Work out the finished part from the listing and answer in its coordinate system (mm). A direction names the side the tool comes from. Coordinates: 2 decimals unless noted, no trailing zeros. Order: outer loops, then holes, each group sorted by start corner. A loop starts at its lowest first (then second) coordinate and runs counter-clockwise, first axis right, second up. Notation, with made-up numbers: (76.25, 24.25) - (108.25, 24.25) arc R12 cw to (108.25, 40.25) - close; hole circle Ø4 at (54.5, 45). An arc over 180 degrees is marked (long way). Answer as a JSON object with one key per item and string values. Group by question number.
1) Find the intervals of material crossed by line 1 along X through (y, z) = (1.5, 14.75); line 2 along X through (y, z) = (7.25, 14.25); line 3 along Y through (x, z) = (15.5, 3), in increasing order.
2) Section B-B (x = 12.5) is taken. Give the vertices of the cut face in (y, z).
3) A tool of negligible diameter and unlimited length cuts with its end or side. For faces 5 (the face through (4.5, 2.2, 19.5)), 6 (the face through (21.6, 14.3, 0.7)), 7 (the face through (14, 13, 14)), from which of +Z, -Z, +X, -X, +Y, -Y can it reach the whole face along a straight path? Write none if from no direction.
4) The mould has two halves that part along Z. Classify faces 1 (the face through (18.7, 7.7, 0.5)), 2 (the face through (2.5, 0.5, 19.5)), 3 (the face through (19.2, 7, 10)), 4 (the face through (7.9, 14.2, 9.9)): released by +Z, released by -Z, zero draft, split by the parting line, or undercut.
5) Each of these flat-tipped pins is pushed along its axis until it touches: P1, Ø2.5, axis at y = 8, z = 6.5, coming from the +X side; P2, Ø4, axis at x = 14, z = 8.5, coming from the +Y side; P3, Ø4, axis at y = 11, z = 18, coming from the -X side; P4, Ø9, axis at x = 11.5, z = 9, coming from the -Y side. Where does it stop, or does it pass through?
Autodesk Inventor part; units mm, degrees
ref_plane "YZ Plane" through (0, 0, 0) normal (1, 0, 0) x (0, 1, 0)
ref_plane "XZ Plane" through (0, 0, 0) normal (0, 1, 0) x (-1, 0, 0)
ref_plane "XY Plane" through (0, 0, 0) normal (0, 0, 1) x (1, 0, 0)
sketch "Base Sketch" plane through (0, 0, 0) normal (0, 0, 1) x (1, 0, 0)
  line L0 (0, 0) -> (5, 0)
  line L1 (5, 0) -> (5, 3)
  line L2 (5, 3) -> (8, 6)
  line L3 (8, 6) -> (19.2, 6)
  line L4 (22.2, 15) -> (0, 15)
  line L5 (0, 15) -> (0, 0)
  line L6 (19.2, 6) -> (19.2, 9)
  line L7 (19.2, 9) -> (22.2, 12)
  line L8 (22.2, 12) -> (22.2, 15)
  dimension "d0" = 45
  dimension "d2" = 5
  dimension "d4" = 11.2
  dimension "d7" = 3
  dimension "d32" = 3
  dimension "d45" = 3
  dimension "d47" = 3
extrude "Profile" add sketch "Base Sketch" along normal blind 20
sketch "CB Slot Sketch" plane through (0, 15, 0) normal (0, 1, 0) x (1, 0, 0)
  line L0 (10, -10) -> (17.2, -10) construction
  line L1 (12.1, -12.1) -> (15.1, -12.1)
  line L2 (15.1, -7.9) -> (12.1, -7.9)
  arc A0 (12.1, -7.9) -> (12.1, -12.1) centre (12.1, -10) ccw
  arc A1 (15.1, -12.1) -> (15.1, -7.9) centre (15.1, -10) ccw
  line L3 (12.1, -10) -> (15.1, -10) construction
  line L4 (12.1, -14.0005) -> (15.1, -14.0005)
  line L5 (15.1, -5.9995) -> (12.1, -5.9995)
  arc A2 (12.1, -5.9995) -> (12.1, -14.0005) centre (12.1, -10) ccw
  arc A3 (15.1, -14.0005) -> (15.1, -5.9995) centre (15.1, -10) ccw
  line L6 (8, 0) -> (19.2, 0) construction
  line L7 (19.2, 0) -> (19.2, -20) construction
  line L8 (8, -20) -> (19.2, -20) construction
  line L9 (8, 0) -> (8, -20) construction
  point P0 (13.6, -10)
  point P1 (10, -10)
  point P2 (8.0995, -10)
  point P3 (13.6, -20)
  point P4 (8, -10)
  dimension "d11" = 4.2
  dimension "d16" = 8.001
  dimension "d24" = 3
extrude "M4 Slot" cut sketch "CB Slot Sketch" against normal through all contours A0 L2 A1 L1
extrude "M4 CB Slot" cut sketch "CB Slot Sketch" against normal blind 4 contours A0 L2 A1 L1 | A2 L5 A3 L4
sketch "Inset Pattern" plane through (0, 0, 0) normal (-1, 0, 0) x (0, 0, 1)
  line L0 (0, 15) -> (0, 0) construction
  line L1 (0, 0) -> (20, 0) construction
  line L2 (20, 15) -> (20, 0) construction
  line L3 (0, 15) -> (20, 15) construction
  line L4 (2.5, 12.5) -> (17.5, 12.5)
  line L5 (17.5, 12.5) -> (17.5, 2.5)
  line L6 (17.5, 2.5) -> (2.5, 2.5)
  line L7 (2.5, 2.5) -> (2.5, 12.5)
  point P0 (17.5, 7.5)
  point P1 (20, 7.5)
  point P2 (10, 12.5)
  point P3 (10, 15)
  dimension "d48" = 15
  dimension "d49" = 10
extrude "Inset" cut sketch "Inset Pattern" against normal blind 0.5
chamfer "Inset Chamfer" distance 0.5 angle 45 4 edges at (0, 12.5, 10) (0, 7.5, 17.5) (0, 7.5, 2.5) (0, 2.5, 10)
chamfer "Edgebreak" distance 1 angle 45 26 edges at (11.1, 15, 20) (11.1, 15, 0) (0, 15, 10) (0, 7.5, 20) (0, 7.5, 0) (0, 0, 10) (2.5, 0, 20) (2.5, 0, 0) (20.7, 10.5, 20) (19.2, 7.5, 20) (13.6, 6, 20) (6.5, 4.5, 20) (5, 1.5, 20) (5, 1.5, 0) (6.5, 4.5, 0) (13.6, 6, 0) (19.2, 7.5, 0) (20.7, 10.5, 0) (19.1005, 15, 10) (13.6, 15, 14.0005) (8.0995, 15, 10) (13.6, 15, 5.9995) (22.2, 13.5, 20) (22.2, 13.5, 0) (22.2, 15, 10) (5, 0, 10)
equation "\"d7\" = d6"
equation "\"d24\" = jawTravel"
equation "\"jawTravel\" = 3"
equation "\"slotLength\" = M4_clearance_hole + jawTravel"
equation "\"M4_clearance_hole\" = 4.2"
equation "\"chamferSize\" = 1"
equation "\"jawThickness\" = 5"
equation "\"topThickness\" = 3"
properties part number "Moving Jaw (M4) Normal" material "ABS Plastic"
Report:
{
 "1": {"line 1": "x = 0 to 5", "line 2": "x = 0.5 to 19.2", "line 3": "y = 6 to 15"},
 "2": {"outline": "(6, 1) - (7, 0) - (14, 0) - (15, 1) - (15, 5) - (14, 6) - (11, 6) - (11, 7.9) - (6, 7.9) - close; (6, 12.1) - (11, 12.1) - (11, 14) - (14, 14) - (15, 15) - (15, 19) - (14, 20) - (7, 20) - (6, 19) - close"},
 "3": {"face 5": "+Z, +X, -Y", "face 6": "-Z, +X, +Y", "face 7": "+Y"},
 "4": {"face 1": "released by -Z", "face 2": "released by +Z", "face 3": "zero draft", "face 4": "undercut"},
 "5": {"P1": "stops at x = 19.45", "P2": "stops at y = 11", "P3": "stops at x = 0", "P4": "stops at y = 5"}
}
